Geometry: see drawing. Coordinates: mm, zero at the bounding-box minimum. A direction names the side the tool comes from. Coordinates: 2 decimals unless noted, no trailing zeros. Loops run counter-clockwise (first coordinate to the right, second up) from the corner with the lowest first, then second, coordinate; pieces in that order, holes last.
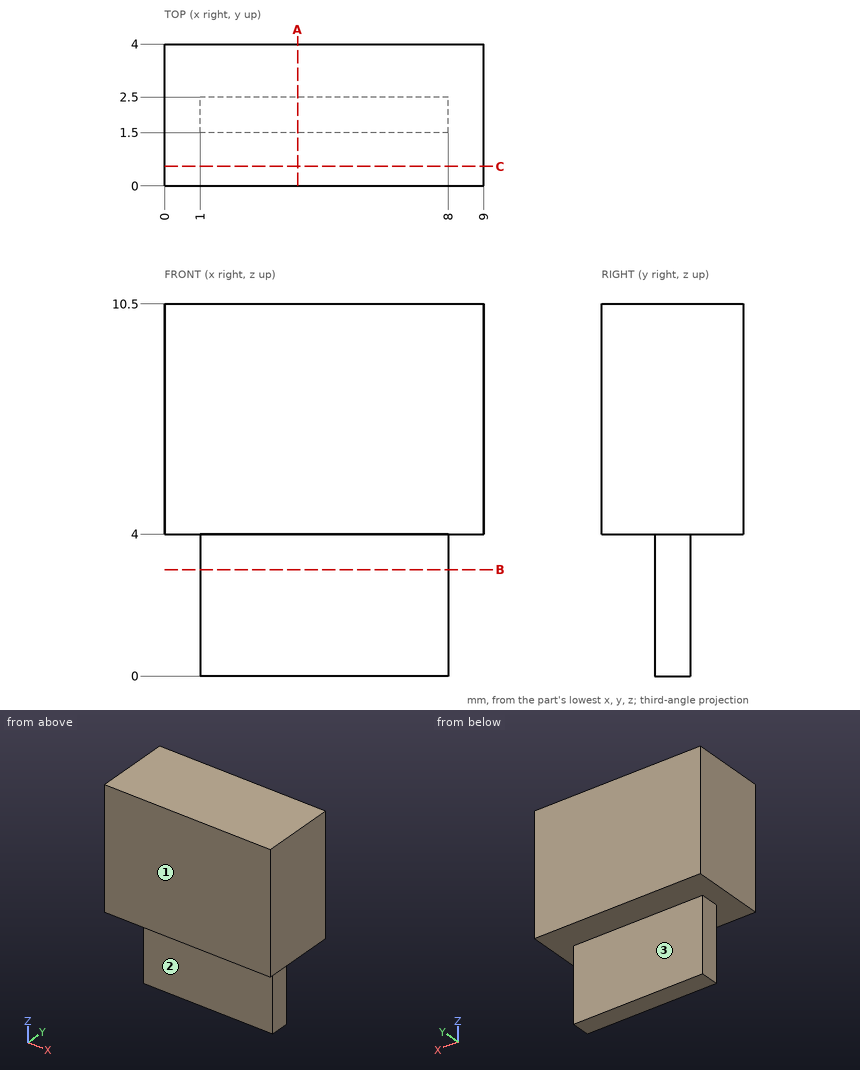
Item 1: Section query A-A (x = 3.75). Output: boundary loops of the cut face in (y, z).
Result:
outline: (0, 4) - (1.5, 4) - (1.5, 0) - (2.5, 0) - (2.5, 4) - (4, 4) - (4, 10.5) - (0, 10.5) - close
Item 2: Reachability of the marked faces 1, 2 and 3 from +Z, -Z, +X, -X, +Y, -Y: full face, straight path, thin tool, end or side. Return the list, or none.
Result:
face 1: +Z, -Z, +X, -X, -Y
face 2: -Z, +X, -X, -Y
face 3: -Z, +X, -X, +Y
Item 3: Contact query for flat-ended pins moving along their axis: P1, Ø0.5, axis at y = 2, z = 1, coming from the +X side; P2, Ø3, axis at x = 4, z = 1, coming from the -Y side; P3, Ø0.8, axis at y = 2, z = 1.5, coming from the -X side. Output: stop coordinate, or through.
Result:
P1: stops at x = 8
P2: stops at y = 1.5
P3: stops at x = 1
Item 4: Section query B-B (z = 3). Output: boundary loops of the cut face in (x, y).
Result:
outline: (1, 1.5) - (8, 1.5) - (8, 2.5) - (1, 2.5) - close
Item 5: Section query C-C (y = 0.55). Output: boundary loops of the cut face in (x, z), then the cut area to 3 significant figures.
Result:
outline: (0, 4) - (9, 4) - (9, 10.5) - (0, 10.5) - close
area: 58.5 mm2
Item 6: Line query: L1, parallel to Z at x = 5.5, y = 1.4; L2, parallel to Y at x = 6.25, z = 1.75; L3, parallel to X at y = 1.6, z = 2.75. Output: solid intervals per line, ascending.
Result:
L1: z = 4 to 10.5
L2: y = 1.5 to 2.5
L3: x = 1 to 8
